Model file for the job. Use its own axes, mm. Face numbers are marked on the shaded views. Give positions to 0.01 mm unless a question says otherwise; leave off trailing zeros. Loops run counter-clockwise (first coordinate to the right, second up) from the corner with the lowest first, then second, coordinate; pieces in that order, holes last. Notation, with made-up numbers: (78, 76) -> (86, 76) arc R20 ccw to (86, 82) -> close; hole circle Ø11 at (68.25, 57). An arc over 180 degrees is marked (long way). Use CSV: the item, a comma, the result in double quotes. Start each with the question number.
(1) Cut at C-C on z = 0. Write the cut outline in (x, y).
(2) Cut at D-D on z = -21. Write the cut outline in (x, y).
(3) Cut at B-B on y = 4.5. State how many separate pieces and enclosed holes the cut face has, then the cut area to 3 significant figures.
(4) Flat gauge pins, fed straight in: pin 1 (5 mm diameter, centred on x = -21, z = 30, fed in from -Y); pin 2 (1.9 mm diameter, centred on x = -3.5, y = 3.5, fed in from +Z); pin 3 (1.9 mm diameter, centred on y = 3.5, z = 3.5, fed in from +X); pin 4 (3 mm diameter, centred on y = 1.5, z = 23.5, fed in from +X) (3 decimals). Where does each tip first touch, or does it go through?
(5) Drill centre lines: probe 1 along X at (y, z) = (3, -15.5); probe 2 along Z at (x, y) = (-15, 6.25); probe 3 along X at (y, z) = (4.5, -31). Where is each one in solid material? Low to high.
(6) Cut at A-A on x = 0. Write the cut outline in (y, z), then the cut area to 3 significant figures.
(7) Pull direction X, two halves, no side cores. Call the marked faces 1, 2 and 3: pulls with the +X half, pulls with the -X half, needs draft (parallel to the pull), parting line crosses it, or undercut.
from build123d import *

# Parameters (mm, degrees)
SKETCH1_R           = 8
SKETCH1_W           = 42
SKETCH1_H           = 60
BOSS_EXTRUDE1_DEPTH = 6.35
SKETCH2_R           = 1.5
SKETCH2_R_2         = 14
CUT_EXTRUDE1_DEPTH  = 49.221597858
SKETCH3_R           = 1.5
CUT_EXTRUDE2_DEPTH  = 49.221597858
FILLET1_R           = 5


with BuildPart() as part:
    # Sketch1 → Boss-Extrude1 (new body)
    with BuildSketch(Plane(origin=(0, 0, 0), x_dir=(1, 0, 0), z_dir=(0, 1, 0))):
        with BuildLine():
            ThreePointArc((-21, -22), (-26.656854249, -35.656854249), (-13, -30))
            Line((-13, -30), (-21, -30))
            Line((-21, -30), (-21, -22))
        make_face()
        with BuildLine():
            Line((-21, -30), (-13, -30))
            ThreePointArc((-13, -30), (-15.343145751, -24.343145751), (-21, -22))
            Line((-21, -22), (-21, -30))
        make_face()
        with BuildLine():
            ThreePointArc((21, -22), (15.343145751, -24.343145751), (13, -30))
            Line((13, -30), (21, -30))
            Line((21, -30), (21, -22))
        make_face()
        with BuildLine():
            Line((21, -30), (13, -30))
            ThreePointArc((13, -30), (21, -38), (29, -30))
            ThreePointArc((29, -30), (26.656854249, -24.343145751), (21, -22))
            Line((21, -22), (21, -30))
        make_face()
        with Locations((21, -30)):
            Circle(SKETCH1_R)
        with Locations((21, 30)):
            Circle(SKETCH1_R)
        with Locations((-21, 30)):
            Circle(SKETCH1_R)
        with Locations((-21, -30)):
            Circle(SKETCH1_R)
        Rectangle(SKETCH1_W, SKETCH1_H)
        with BuildLine():
            ThreePointArc((13, 30), (15.343145751, 24.343145751), (21, 22))
            Line((21, 22), (21, 30))
            Line((21, 30), (13, 30))
        make_face()
        with BuildLine():
            Line((21, 30), (21, 22))
            ThreePointArc((21, 22), (26.656854249, 24.343145751), (29, 30))
            ThreePointArc((29, 30), (21, 38), (13, 30))
            Line((13, 30), (21, 30))
        make_face()
        with BuildLine():
            ThreePointArc((-13, 30), (-26.656854249, 35.656854249), (-21, 22))
            Line((-21, 22), (-21, 30))
            Line((-21, 30), (-13, 30))
        make_face()
        with BuildLine():
            Line((-21, 30), (-21, 22))
            ThreePointArc((-21, 22), (-15.343145751, 24.343145751), (-13, 30))
            Line((-13, 30), (-21, 30))
        make_face()
    extrude(amount=BOSS_EXTRUDE1_DEPTH)

    # Sketch2 → Cut-Extrude1 (cut, through all)
    with BuildSketch(Plane(origin=(0, 6.35, 0), x_dir=(1, 0, 0), z_dir=(0, 1, 0))):
        with Locations(Location((-15.5, -15.5, 0), (0, 0, 270))):
            Circle(SKETCH2_R)
        with Locations(Location((15.5, -15.5, 0), (0, 0, 270))):
            Circle(SKETCH2_R)
        with Locations(Location((15.5, 15.5, 0), (0, 0, 270))):
            Circle(SKETCH2_R)
        with Locations(Location((-15.5, 15.5, 0), (0, 0, 270))):
            Circle(SKETCH2_R)
        with Locations(Location((0, 0, 0), (0, 0, 270))):
            Circle(SKETCH2_R_2)
    extrude(amount=-CUT_EXTRUDE1_DEPTH, mode=Mode.SUBTRACT)

    # Sketch3 → Cut-Extrude2 (cut, through all)
    with BuildSketch(Plane(origin=(0, 6.35, 0), x_dir=(1, 0, 0), z_dir=(0, 1, 0))):
        with Locations(Location((-21, 30, 0), (0, 0, 270))):
            Circle(SKETCH3_R)
        with Locations(Location((21, 30, 0), (0, 0, 270))):
            Circle(SKETCH3_R)
        with Locations(Location((21, -30, 0), (0, 0, 270))):
            Circle(SKETCH3_R)
        with Locations(Location((-21, -30, 0), (0, 0, 270))):
            Circle(SKETCH3_R)
    extrude(amount=-CUT_EXTRUDE2_DEPTH, mode=Mode.SUBTRACT)

    # Fillet1
    fillet1_edges = [part.edges().sort_by_distance(p)[0] for p in [
        (13, 3.175, 30),
        (-13, 3.175, 30),
        (-21, 3.175, 22),
        (-21, 3.175, -22),
        (-13, 3.175, -30),
        (13, 3.175, -30),
        (21, 3.175, -22),
        (21, 3.175, 22),
    ]]
    fillet(fillet1_edges, radius=FILLET1_R)


solid = part.part
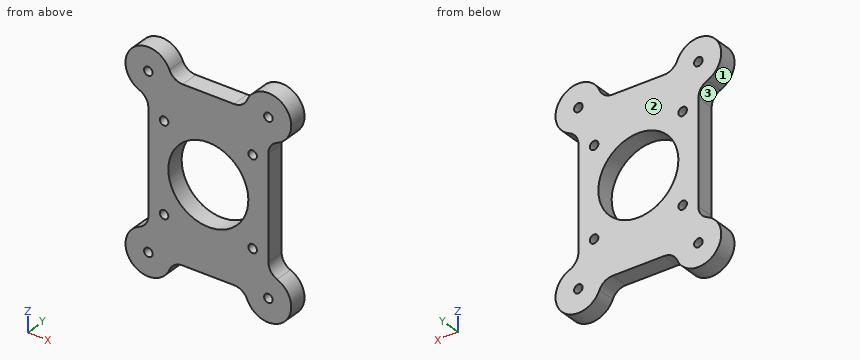
Check result:
1,outline,"(-21, 0) -> (-14, 0) -> (-14, 6.35) -> (-21, 6.35) -> close; (14, 0) -> (21, 0) -> (21, 6.35) -> (14, 6.35) -> close"
2,outline,"(-22, 0) -> (22, 0) -> (22, 6.35) -> (-22, 6.35) -> close"
3,separate pieces,"1"
3,enclosed holes,"9"
3,area,"2,470 mm²"
4,pin 1,"y = 0"
4,pin 2,"z = 30"
4,pin 3,"x = 21"
4,pin 4,"x = 27.245"
5,probe 1,"-21 to -17, -14 to 14, 17 to 21"
5,probe 2,"-35.29 to -16.91, -14.09 to 14.09, 16.91 to 35.29"
5,probe 3,"-28.94 to -22.12, -19.88 to -12, 12 to 19.88, 22.12 to 28.94"
6,outline,"(0, -30) -> (6.35, -30) -> (6.35, -14) -> (0, -14) -> close; (0, 14) -> (6.35, 14) -> (6.35, 30) -> (0, 30) -> close"
6,area,"203 mm²"
7,face 1,"undercut"
7,face 2,"needs draft"
7,face 3,"pulls with the -X half"
